Model file for the job. Use its own axes, mm. Give positions to 0.01 mm unless a question says otherwise; leave off trailing zeros. Loops run counter-clockwise (first coordinate to the right, second up) from the corner with the lowest first, then second, coordinate; pieces in that order, holes last. Notation, with made-up numbers: (20, 75) - (35, 75) arc R19 cw to (35, 82) - close; hole circle Ø10 at (72.25, 64.5). An arc over 180 degrees is marked (long way). Answer as CSV lines item,"result". Start each with the question number.
Item 1: Drill centre lines: L1, parallel to X at y = 2.2, z = 0 (3 decimals); L2, parallel to Z at x = 10, y = 1.55 (3 decimals); L3, parallel to X at y = 1.5, z = 1.25. Where is each one in solid material? Low to high. Write a range as from..to.
Item 2: Pin check, flat tip, straight feed: pin 1 (1.7 mm diameter, centred on x = 50, z = 0, fed in from -Y). Stop position of the tip, or through.
Item 3: Saw through at A-A on z = 0. Give the cut face in (x, y) (3 decimals).
Item 4: Saw through at B-B on x = 10. Give the cut face in (y, z) (3 decimals), plus the area to 4 significant figures.
from build123d import *

# Parameters (mm, degrees)
SKETCH1_W           = 100
SKETCH1_H           = 15
BOSS_EXTRUDE1_DEPTH = 3
SKETCH2_R           = 1
CUT_EXTRUDE1_DEPTH  = 10
SKETCH3_R           = 2.5
CUT_EXTRUDE2_DEPTH  = 10
CUT_EXTRUDE3_DEPTH  = 10
FILLET1_R           = 5
FILLET2_R           = 1
SKETCH7_W           = 15
SKETCH7_H           = 3
BOSS_EXTRUDE2_DEPTH = 20
SKETCH8_W           = 41.116503549
SKETCH8_H           = 15
CUT_EXTRUDE6_DEPTH  = 20
SKETCH9_R           = 1.425
CUT_EXTRUDE7_DEPTH  = 20


with BuildPart() as part:
    # Sketch1 → Boss-Extrude1 (new body)
    with BuildSketch(Plane(origin=(0, 0, 0), x_dir=(1, 0, 0), z_dir=(0, 1, 0))):
        Rectangle(SKETCH1_W, SKETCH1_H)
    extrude(amount=BOSS_EXTRUDE1_DEPTH)

    # Sketch2 → Cut-Extrude1 (cut)
    with BuildSketch(Plane(origin=(0, 3, 0), x_dir=(1, 0, 0), z_dir=(0, 1, 0))):
        with Locations((-28.87, 0)):
            Circle(SKETCH2_R)
        with Locations((-42, 0)):
            Circle(SKETCH2_R)
    extrude(amount=-CUT_EXTRUDE1_DEPTH, mode=Mode.SUBTRACT)

    # Sketch3 → Cut-Extrude2 (cut)
    with BuildSketch(Plane.XZ):
        with Locations((-35.434103263, -0.006545742)):
            Circle(SKETCH3_R)
    extrude(amount=-CUT_EXTRUDE2_DEPTH, mode=Mode.SUBTRACT)

    # Sketch4 → Cut-Extrude3 (cut)
    with BuildSketch(Plane(origin=(0, 0, 0), x_dir=(-1, 0, 0), z_dir=(0, -1, 0))):
        with BuildLine():
            Line((50, 1.885031535), (50, 7.5))
            Line((50, 7.5), (39.062958866, 7.5))
            Line((39.062958866, 7.5), (41.762759664, 3.577599022))
            ThreePointArc((41.762759664, 3.577599022), (42.595166406, 2.79306797), (43.676751147, 2.42082557))
            Line((43.676751147, 2.42082557), (50, 1.885031535))
        make_face()
    cut_extrude3 = extrude(amount=-CUT_EXTRUDE3_DEPTH, mode=Mode.SUBTRACT)

    # Mirror1: Cut-Extrude3 across plane
    add(cut_extrude3.mirror(Plane.XY), mode=Mode.SUBTRACT)

    # Fillet1
    fillet1_edges = [part.edges().sort_by_distance(p)[0] for p in [
        (-39.062958866, 1.5, -7.5),
        (-39.062958866, 1.5, 7.5),
    ]]
    fillet(fillet1_edges, radius=FILLET1_R)

    # Fillet2
    fillet2_edges = [part.edges().sort_by_distance(p)[0] for p in [
        (-50, 1.5, -1.885031535),
        (-50, 1.5, 1.885031535),
    ]]
    fillet(fillet2_edges, radius=FILLET2_R)

    # Sketch7 → Boss-Extrude2 (add)
    with BuildSketch(Plane(origin=(50, 0, 0), x_dir=(0, 0, -1), z_dir=(1, 0, 0))):
        with Locations((0, 1.5)):
            Rectangle(SKETCH7_W, SKETCH7_H)
    extrude(amount=BOSS_EXTRUDE2_DEPTH)

    # Sketch8 → Cut-Extrude6 (cut)
    with BuildSketch(Plane(origin=(0, 3, 0), x_dir=(1, 0, 0), z_dir=(0, 1, 0))):
        with Locations((-40.558251775, 0)):
            Rectangle(SKETCH8_W, SKETCH8_H)
    extrude(amount=-CUT_EXTRUDE6_DEPTH, mode=Mode.SUBTRACT)

    # Sketch9 → Cut-Extrude7 (cut)
    with BuildSketch(Plane(origin=(0, 3, 0), x_dir=(1, 0, 0), z_dir=(0, 1, 0))):
        with Locations((50, 0)):
            Circle(SKETCH9_R)
        with Locations((10, 0)):
            Circle(SKETCH9_R)
    extrude(amount=-CUT_EXTRUDE7_DEPTH, mode=Mode.SUBTRACT)


solid = part.part
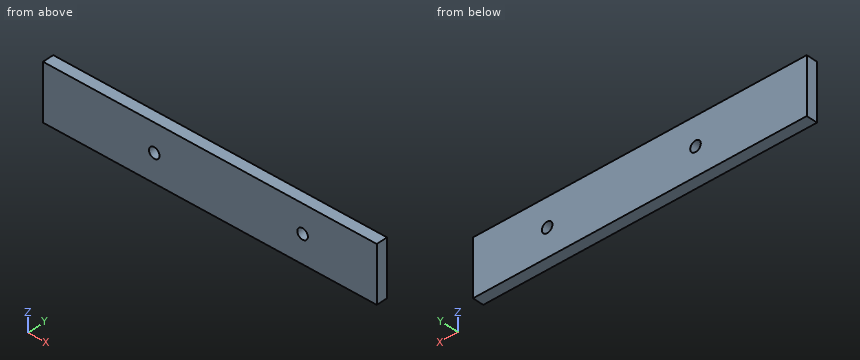
Responses:
1,L1,"-20..8.575, 11.425..48.575, 51.425..70"
1,L2,"-7.5..-1.425, 1.425..7.5"
1,L3,"-20..9.32, 10.68..49.32, 50.68..70"
2,pin 1,"through"
3,outline,"(-20, 0) - (8.575, 0) - (8.575, 3) - (-20, 3) - close; (11.425, 0) - (48.575, 0) - (48.575, 3) - (11.425, 3) - close; (51.425, 0) - (70, 0) - (70, 3) - (51.425, 3) - close"
4,outline,"(0, -7.5) - (3, -7.5) - (3, -1.425) - (0, -1.425) - close; (0, 1.425) - (3, 1.425) - (3, 7.5) - (0, 7.5) - close"
4,area,"36.45 mm2"
